The model under review builds one solid part; all positions refer to its coordinate system, in mm. Face numbers are marked on the shaded views. Give positions to 0.01 mm unless a question says otherwise; leave off trailing zeros. Loops run counter-clockwise (first coordinate to the right, second up) from the corner with the lowest first, then second, coordinate; pieces in that order, holes last. Notation, with made-up numbers: M 12.25,5.25 L 18.25,5.25 A24 cw 18.25,33.25 Z; hole C 51.5,41.5 d5. An arc over 180 degrees is marked long. Return JSON: item names as keys, results as strings. Group by question number.
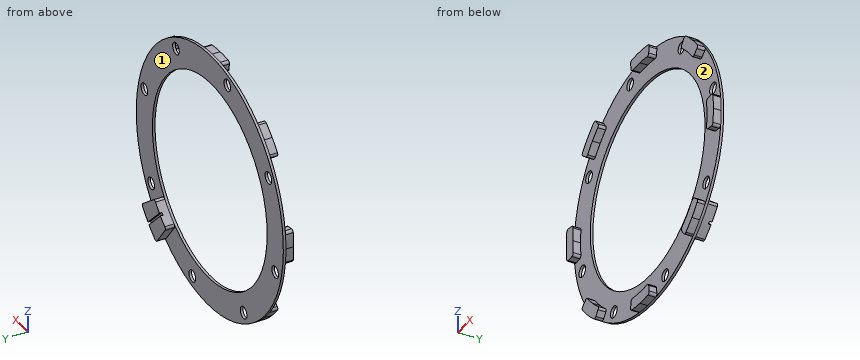
```python
from build123d import *
from build123d.topology import SkipClean

# Parameters (mm, degrees)
SKETCH_1_R               = 50
SKETCH_1_R_2             = 39
EXTRUDE_1_DEPTH          = 1
SKETCH_2_R               = 2.25
CUT_EXTRUDE_1_DEPTH      = 2
EXTRUDE_START            = 3
EXTRUDE_2_DEPTH          = 3
FILLET_1_R               = 1
PATTERN_CIRCULAR_1_COUNT = 8
EXTRUDE_3_DEPTH          = 3.6
FILLET_2_R               = 1
FILLET_3_R               = 1
CUT_EXTRUDE_2_DEPTH      = 1


with BuildPart() as part:
    # 草图1 → 凸台-拉伸1 (new body)
    with BuildSketch(Plane(origin=(0, 0, 0), x_dir=(1, 0, 0), z_dir=(0, 1, 0))):
        with Locations(Location((0, 0, 0), (0, 0, 270))):
            Circle(SKETCH_1_R)
        with Locations(Location((0, 0, 0), (0, 0, 270))):
            Circle(SKETCH_1_R_2, mode=Mode.SUBTRACT)
    extrude(amount=EXTRUDE_1_DEPTH)

    # 草图2 → 切除-拉伸1 (cut)
    with BuildSketch(Plane(origin=(0, 1, 0), x_dir=(1, 0, 0), z_dir=(0, 1, 0))):
        with Locations(Location((11.905676075, 44.432588009, 0), (0, 0, 270))):
            Circle(SKETCH_2_R)
        with Locations(Location((-23, 39.837168574, 0), (0, 0, 270))):
            Circle(SKETCH_2_R)
        with Locations(Location((39.837168574, 23, 0), (0, 0, 270))):
            Circle(SKETCH_2_R)
        with Locations(Location((44.432588009, -11.905676075, 0), (0, 0, 270))):
            Circle(SKETCH_2_R)
        with Locations(Location((23, -39.837168574, 0), (0, 0, 270))):
            Circle(SKETCH_2_R)
        with Locations(Location((-11.905676075, -44.432588009, 0), (0, 0, 270))):
            Circle(SKETCH_2_R)
        with Locations(Location((-39.837168574, -23, 0), (0, 0, 270))):
            Circle(SKETCH_2_R)
        with Locations(Location((-44.432588009, 11.905676075, 0), (0, 0, 270))):
            Circle(SKETCH_2_R)
    extrude(amount=-CUT_EXTRUDE_1_DEPTH, mode=Mode.SUBTRACT)

    # 草图3 → 凸台-拉伸2 (add)
    with BuildSketch(Plane.XZ.offset(EXTRUDE_START)):
        with BuildLine():
            ThreePointArc((-5.873079204, 45.220205005), (-2.942673256, 45.504952193), (0, 45.6))
            Line((0, 45.6), (0, 50))
            ThreePointArc((0, 50), (-3.226615413, 49.895780914), (-6.439779829, 49.583558119))
            Line((-6.439779829, 49.583558119), (-5.873079204, 45.220205005))
        make_face()
        with BuildLine():
            Line((0, 50), (0, 45.6))
            ThreePointArc((0, 45.6), (2.942673256, 45.504952193), (5.873079204, 45.220205005))
            Line((5.873079204, 45.220205005), (6.439779829, 49.583558119))
            ThreePointArc((6.439779829, 49.583558119), (3.226615413, 49.895780914), (0, 50))
        make_face()
    extrude_2 = extrude(amount=-EXTRUDE_2_DEPTH)

    # 圆角1
    fillet_1_edges = [part.edges().sort_by_distance(p)[0] for p in [
        (-5.873079204, -1.5, 45.220205005),
        (5.873079204, -1.5, 45.220205005),
    ]]
    fillet(fillet_1_edges, radius=FILLET_1_R)

    # 阵列(圆周)1: 凸台-拉伸2 ×8 about axis
    with SkipClean():  # the faces are left unmerged after this step: merging them gives an invalid solid
        pattern_circular_1_axis = Axis((0, 0, 0), (0, 1, 0))
        for i in range(1, PATTERN_CIRCULAR_1_COUNT):
            add(extrude_2.rotate(pattern_circular_1_axis, i * 360 / PATTERN_CIRCULAR_1_COUNT))

    # 草图4 → 凸台-拉伸3 (add)
    with SkipClean():  # the faces are left unmerged after this step: merging them gives an invalid solid
        with BuildSketch(Plane(origin=(0, 1, 0), x_dir=(1, 0, 0), z_dir=(0, 1, 0))):
            with BuildLine():
                ThreePointArc((23.470785903, 31.146784892), (27.577164466, 27.577164466), (31.146784892, 23.470785903))
                Line((31.146784892, 23.470785903), (39.931775502, 30.090751158))
                ThreePointArc((39.931775502, 30.090751158), (35.355339059, 35.355339059), (30.090751158, 39.931775502))
                Line((30.090751158, 39.931775502), (23.470785903, 31.146784892))
            make_face()
        extrude(amount=EXTRUDE_3_DEPTH)

    # 圆角2
    # the kernel refuses this fillet: 1 mm, written as the material it takes off along each edge
    with BuildSketch(Plane(origin=(30.090751158, 1, -39.931775502), x_dir=(0.7924526369681321, 0, 0.6099334538802196), z_dir=(0, 1, 0))) as fillet_2_piece_1:
        with BuildLine():
            CenterArc((1.010256684, -0.999947932), FILLET_2_R, 89.415308597, 91.169382806)
            Line((0.010308753, -1.010152545), (0, 0))
            ThreePointArc((0, 0), (0.510230649, 0.002603421), (1.020461297, 0))
        make_face()
    extrude(amount=6.151153243, mode=Mode.SUBTRACT)
    with BuildSketch(Plane(origin=(23.470785903, 1, -31.146784892), x_dir=(0.791049828797745, 0, 0.6117517211737605), z_dir=(0, 1, 0))) as fillet_2_piece_2:
        with BuildLine():
            CenterArc((0.98757717, 0.99992186), FILLET_2_R, 180.716271869, 88.567456262)
            Line((-0.01234469, 0.987420883), (0, 0))
            ThreePointArc((0, 0), (0.487538096, 0.00304747), (0.975076193, 0))
        make_face()
    extrude(amount=6.068745116, mode=Mode.SUBTRACT)
    with BuildSketch(Plane(origin=(31.146784892, 1, -23.470785903), x_dir=(-0.611751721173858, 0, -0.7910498287976696), z_dir=(0, 1, 0))) as fillet_2_piece_3:
        with BuildLine():
            CenterArc((0.98757717, -0.99992186), FILLET_2_R, 90.716271869, 88.567456262)
            Line((-0.01234469, -0.987420883), (0, 0))
            ThreePointArc((0, 0), (0.487538096, -0.00304747), (0.975076193, 0))
        make_face()
    extrude(amount=6.068745116, mode=Mode.SUBTRACT)
    with BuildSketch(Plane(origin=(39.931775502, 1, -30.090751158), x_dir=(-0.6099334538803046, 0, -0.7924526369680664), z_dir=(0, 1, 0))) as fillet_2_piece_4:
        with BuildLine():
            CenterArc((1.010256684, 0.999947932), FILLET_2_R, 179.415308597, 91.169382806)
            Line((0.010308753, 1.010152545), (0, 0))
            ThreePointArc((0, 0), (0.510230649, -0.002603421), (1.020461297, 0))
        make_face()
    extrude(amount=6.151153243, mode=Mode.SUBTRACT)

    # 圆角3
    # the kernel refuses this fillet: 1 mm, written as the material it takes off along each edge
    with BuildSketch(Plane(origin=(5.873079204, -5.473172877, -45.220205005), x_dir=(-0.9929960778530438, 0, -0.11814732061486549), z_dir=(0, 1, 0)), Plane(origin=(-27.822619474, -5.473172877, -36.128407737), x_dir=(-0.7856970319273249, 0, 0.6186114887557392), z_dir=(0, 1, 0)), Plane(origin=(-45.220205005, -5.473172877, -5.873079204), x_dir=(-0.11814732061486613, 0, 0.9929960778530437), z_dir=(0, 1, 0)), Plane(origin=(-36.128407737, -5.473172877, 27.822619474), x_dir=(0.6186114887557375, 0, 0.7856970319273263), z_dir=(0, 1, 0)), Plane(origin=(27.822619474, -5.473172877, 36.128407737), x_dir=(0.7856970319273222, 0, -0.6186114887557427), z_dir=(0, 1, 0)), Plane(origin=(45.220205005, -5.473172877, 5.873079204), x_dir=(0.11814732061486592, 0, -0.9929960778530437), z_dir=(0, 1, 0)), Plane(origin=(36.128407737, -5.473172877, -27.822619474), x_dir=(-0.6186114887557427, 0, -0.7856970319273222), z_dir=(0, 1, 0))) as fillet_3_piece_1:
        with BuildLine():
            CenterArc((0.989327342, -0.999942429), FILLET_3_R, 90.614808775, 88.770382449)
            Line((-0.010615087, -0.989212198), (0, 0))
            ThreePointArc((0, 0), (0.489298555, -0.002625219), (0.978597111, 0))
        make_face()
    extrude(amount=5.473172877, mode=Mode.SUBTRACT)
    with BuildSketch(Plane(origin=(-5.873079204, -5.473172877, -45.220205005), x_dir=(-0.1287955965775636, 0, -0.9916711623830904), z_dir=(0, 1, 0)), Plane(origin=(-36.128407737, -5.473172877, -27.822619474), x_dir=(-0.7922896433551908, 0, -0.6101451639012675), z_dir=(0, 1, 0)), Plane(origin=(-45.220205005, -5.473172877, 5.873079204), x_dir=(-0.9916711623830903, 0, 0.12879559657756398), z_dir=(0, 1, 0)), Plane(origin=(-27.822619474, -5.473172877, 36.128407737), x_dir=(-0.6101451639012675, 0, 0.7922896433551908), z_dir=(0, 1, 0)), Plane(origin=(36.128407737, -5.473172877, 27.822619474), x_dir=(0.7922896433551925, 0, 0.6101451639012652), z_dir=(0, 1, 0)), Plane(origin=(45.220205005, -5.473172877, -5.873079204), x_dir=(0.9916711623830904, 0, -0.1287955965775636), z_dir=(0, 1, 0)), Plane(origin=(27.822619474, -5.473172877, -36.128407737), x_dir=(0.6101451639012653, 0, -0.7922896433551926), z_dir=(0, 1, 0))) as fillet_3_piece_2:
        with BuildLine():
            CenterArc((0.989269151, -1), FILLET_3_R, 90, 88.770382449)
            ThreePointArc((-0.010500574, -0.978540773), (-0.002625219, -0.489298555), (0, 0))
            Line((0, 0), (0.989269151, 0))
        make_face()
    extrude(amount=5.473172877, mode=Mode.SUBTRACT)
    with BuildSketch(Plane(origin=(-6.439779829, -5.551153243, -49.583558119), x_dir=(0.9929338368493981, 0, -0.1186692699882022), z_dir=(0, 1, 0)), Plane(origin=(6.439779829, -5.551153243, 49.583558119), x_dir=(-0.9929338368493983, 0, 0.1186692699882015), z_dir=(0, 1, 0)), Plane(origin=(39.614482168, -5.551153243, 30.507258195), x_dir=(-0.6181984037786714, 0, 0.7860220948329013), z_dir=(0, 1, 0)), Plane(origin=(49.583558119, -5.551153243, -6.439779829), x_dir=(0.11866926998820088, 0, 0.9929338368493983), z_dir=(0, 1, 0)), Plane(origin=(30.507258195, -5.551153243, -39.614482168), x_dir=(0.7860220948329028, 0, 0.6181984037786699), z_dir=(0, 1, 0))) as fillet_3_piece_3:
        with BuildLine():
            CenterArc((1.010256684, -0.999947932), FILLET_3_R, 89.415308597, 91.169382806)
            Line((0.010308753, -1.010152545), (0, 0))
            ThreePointArc((0, 0), (0.510230649, 0.002603421), (1.020461297, 0))
        make_face()
    extrude(amount=5.551153243, mode=Mode.SUBTRACT)
    with BuildSketch(Plane(origin=(6.439779829, -5.551153243, -49.583558119), x_dir=(-0.9929338368493981, 0, -0.1186692699882022), z_dir=(0, 1, 0)), Plane(origin=(30.507258195, -5.551153243, 39.614482168), x_dir=(0.7860220948329047, 0, -0.6181984037786672), z_dir=(0, 1, 0)), Plane(origin=(49.583558119, -5.551153243, 6.439779829), x_dir=(0.11866926998820333, 0, -0.992933836849398), z_dir=(0, 1, 0)), Plane(origin=(39.614482168, -5.551153243, -30.507258195), x_dir=(-0.6181984037786714, 0, -0.7860220948329013), z_dir=(0, 1, 0))) as fillet_3_piece_4:
        with BuildLine():
            CenterArc((1.010256684, 0.999947932), FILLET_3_R, 179.415308597, 91.169382806)
            Line((0.010308753, 1.010152545), (0, 0))
            ThreePointArc((0, 0), (0.510230649, -0.002603421), (1.020461297, 0))
        make_face()
    extrude(amount=5.551153243, mode=Mode.SUBTRACT)
    with BuildSketch(Plane(origin=(-39.614482168, -5.551153243, -30.507258195), x_dir=(0.7922896433551889, 0, 0.61014516390127), z_dir=(0, 1, 0)), Plane(origin=(-49.583558119, -5.551153243, 6.439779829), x_dir=(0.9916711623830904, 0, -0.12879559657756223), z_dir=(0, 1, 0)), Plane(origin=(-30.507258195, -5.551153243, 39.614482168), x_dir=(0.6101451639012682, 0, -0.7922896433551903), z_dir=(0, 1, 0))) as fillet_3_piece_5:
        with BuildLine():
            CenterArc((1.010205144, 1), FILLET_3_R, 178.830617194, 91.169382806)
            ThreePointArc((0.010413413, 1.020408163), (0.002603421, 0.510230649), (0, 0))
            Line((0, 0), (1.010205144, 0))
        make_face()
    extrude(amount=5.551153243, mode=Mode.SUBTRACT)
    with BuildSketch(Plane(origin=(-30.507258195, -5.551153243, -39.614482168), x_dir=(0.6101451639012663, 0, 0.7922896433551917), z_dir=(0, 1, 0)), Plane(origin=(-49.583558119, -5.551153243, -6.439779829), x_dir=(0.9916711623830905, 0, 0.1287955965775631), z_dir=(0, 1, 0)), Plane(origin=(-39.614482168, -5.551153243, 30.507258195), x_dir=(0.7922896433551917, 0, -0.6101451639012663), z_dir=(0, 1, 0)), Plane(origin=(-6.439779829, -5.551153243, 49.583558119), x_dir=(0.1287955965775631, 0, -0.9916711623830905), z_dir=(0, 1, 0))) as fillet_3_piece_6:
        with BuildLine():
            CenterArc((1.010205144, -1), FILLET_3_R, 90, 91.169382806)
            ThreePointArc((0.010413413, -1.020408163), (0.002603421, -0.510230649), (0, 0))
            Line((0, 0), (1.010205144, 0))
        make_face()
    extrude(amount=5.551153243, mode=Mode.SUBTRACT)

    # 草图5 → 切除-拉伸2 (cut)
    with BuildSketch(Plane(origin=(0, 4.6, 0), x_dir=(1, 0, 0), z_dir=(0, 1, 0))):
        Polygon((36.054313611, 36.761420392), (36.761420392, 36.054313611), (25.110197925, 24.403091144), (24.403091144, 25.110197925), align=None)
    extrude(amount=-CUT_EXTRUDE_2_DEPTH, mode=Mode.SUBTRACT)


solid = part.part
```
(1) Add section D-D (z = 27). Write out the cut boundary in (x, y).
(2) Mouldability with a two-part tool opening along X and no side actions: class the marked faces 1 and 2 as released by +X, released by -X, zero draft, split by the parting line, or undercut.
(3) Add section C-C (x = -23). Write out the cut boundary in (y, z), and give its area (3 significant figures).
(4) Add section A-A (z = -1.5). Write out the cut boundary in (x, y).
(5) Add section B-B (x = -3.5). Write out the cut boundary in (y, z), and give its area (3 significant figures).
(6) For pin 1 (7 mm diameter, centred on x = 23, z = 39.84, fed in from -Y); pin 2 (6 mm diameter, centred on x = -11.91, z = 44.43, fed in from +Y), all flat-tipped, find the tip position at first contact; note any pin that passes through.
(7) For probe 1 along Z at (x, y) = (-1, -1.25); probe 2 along Y at (x, z) = (-15, 45.5); probe 3 along X at (y, z) = (0.5, -28), list the stretches that pass through material, from the lowest coordinate up.
Verdict:
{
 "1": {"outline": "M -42.08,0 L -28.14,0 L -28.14,1 L -42.08,1 Z; M 28.14,0 L 42.08,0 L 42.08,1 L 28.14,1 Z"},
 "2": {"face 1": "zero draft", "face 2": "undercut"},
 "3": {"outline": "M 0,-44.4 L 1,-44.4 L 1,-42.09 L 0,-42.09 Z; M 0,-37.59 L 1,-37.59 L 1,-31.5 L 0,-31.5 Z; M 0,31.5 L 1,31.5 L 1,44.4 L 0,44.4 Z", "area": "21.3 mm²"},
 "4": {"outline": "M -49.98,-3 L -45.58,-3 L -45.58,0 L -38.97,0 L -38.97,1 L -49.98,1 Z; M 38.97,0 L 45.58,0 L 45.58,-3 L 49.98,-3 L 49.98,1 L 38.97,1 Z"},
 "5": {"outline": "M -3,-49.88 L 1,-49.88 L 1,-38.84 L 0,-38.84 L 0,-45.47 L -3,-45.47 Z; M -3,45.47 L 0,45.47 L 0,38.84 L 1,38.84 L 1,49.88 L -3,49.88 Z", "area": "48.5 mm²"},
 "6": {"pin 1": "stops at y = 0", "pin 2": "stops at y = 1"},
 "7": {"probe 1": "z = -49.99 to -45.59, 45.59 to 49.99", "probe 2": "y = 0 to 1", "probe 3": "x = -41.42 to -27.15, 27.15 to 41.42"}
}
